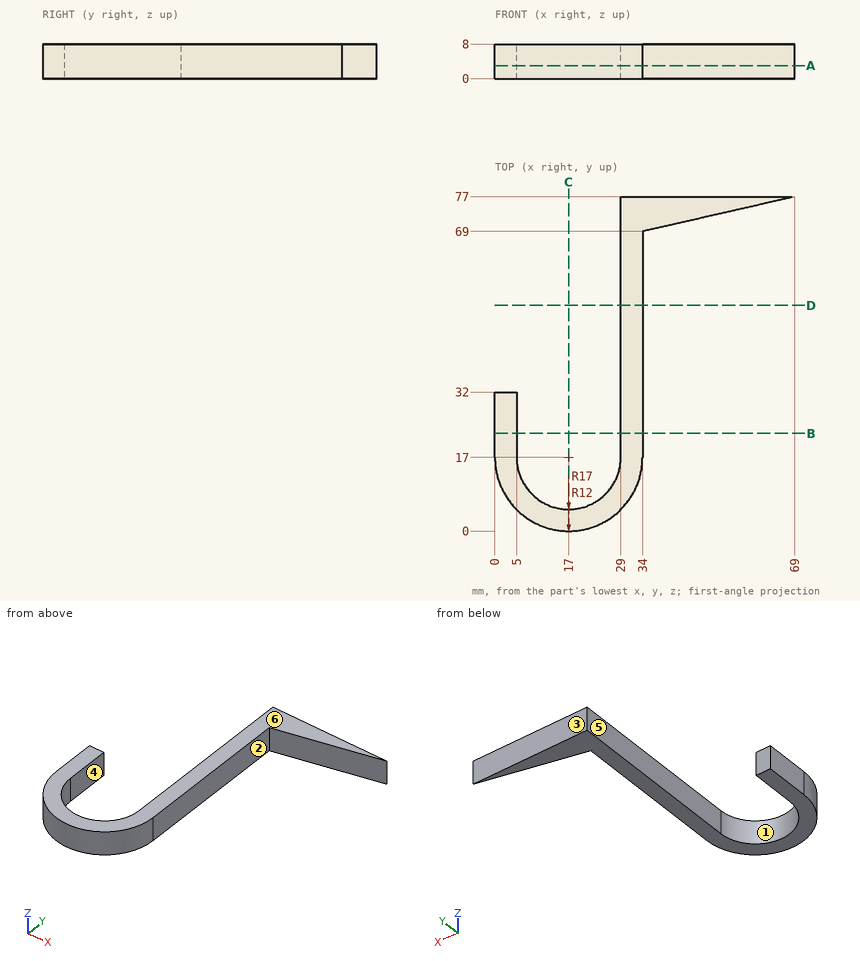
The figure shows three views and two pictorial views of one solid part (mm, origin at its lowest corner). Answer the questions. A direction names the side the tool comes from. Give positions to 0.01 mm unless a question says otherwise; leave off trailing zeros. Write each loop counter-clockwise with the first axis right and the second up, starting at its lowest first coordinate (ties: lowest second). Pieces come first, ordered by that corner, then holes. Notation, with made-up numbers: (32.25, 74) - (56.25, 74) arc R27 cw to (56.25, 92) - close; hole circle Ø11 at (-31.5, 36.5). An arc over 180 degrees is marked (long way). Use CSV: the item, a comma, the result in double quotes. Start each with the question number.
Item 1: Consider line 1 (X direction, y = 46, z = 3); line 2 (X direction, y = 8, z = 3.25); line 3 (X direction, y = 9, z = 4.25). Determine where each line is inside the solid, lowest interval first.
Item 2: The part is cut by section D-D, the plane y = 52. Give the vertices of the cut face in (x, z), and give its area (3 significant figures).
Item 3: The mould has two halves that part along X. Classify the marked faces 1, 2, 3 and 4: pulls with the +X half, pulls with the -X half, needs draft (parallel to the pull), parting line crosses it, or undercut.
Item 4: The part is cut by section C-C, the plane x = 17. Give the vertices of the cut face in (y, z).
Item 5: For the marked faces 5 and 6, determine the directions among +Z, -Z, +X, -X, +Y, -Y from which every point of the face is accessible in a straight line to the end or side of a thin tool.
Item 6: The part is cut by section A-A, the plane z = 3. Give the vertices of the cut face in (x, y).
Item 7: Flat-ended cylindrical pins translate along their axes: P1, Ø3, axis at y = 14, z = 6, coming from the -X side; P2, Ø2.5, axis at y = 48, z = 3, coming from the +X side; P3, Ø1.5, axis at x = 9.5, z = 4, coming from the -Y side. Find the tip coordinate at first contact, or state that the pin passes through.
Item 8: The part is cut by section B-B, the plane y = 22.5. Give the vertices of the cut face in (x, z).
Taken from the geometry:
1,line 1,"29 to 34"
1,line 2,"2.58 to 9.06, 24.94 to 31.42"
1,line 3,"2 to 8.06, 25.94 to 32"
2,outline,"(29, 0) - (34, 0) - (34, 8) - (29, 8) - close"
2,area,"40.0 mm2"
3,face 1,"undercut"
3,face 2,"pulls with the +X half"
3,face 3,"needs draft"
3,face 4,"undercut"
4,outline,"(0, 0) - (5, 0) - (5, 8) - (0, 8) - close"
5,face 5,"+Z, -Z, +Y"
5,face 6,"+Z, +X, -X, +Y, -Y"
6,outline,"(0, 17) arc R17 ccw to (34, 17) - (34, 69) - (69, 77) - (29, 77) - (29, 17) arc R12 cw to (5, 17) - (5, 32) - (0, 32) - close"
7,P1,"x = 0.07"
7,P2,"x = 34"
7,P3,"y = 1.4"
8,outline,"(0, 0) - (5, 0) - (5, 8) - (0, 8) - close; (29, 0) - (34, 0) - (34, 8) - (29, 8) - close"
